Autodesk Inventor part; units mm, degrees
ref_plane "YZ Plane" through (0, 0, 0) normal (1, 0, 0) x (0, 1, 0)
ref_plane "XZ Plane" through (0, 0, 0) normal (0, 1, 0) x (-1, 0, 0)
ref_plane "XY Plane" through (0, 0, 0) normal (0, 0, 1) x (1, 0, 0)
sketch "Sketch1" plane through (0, 0, 0) normal (0, 0, 1) x (1, 0, 0)
  circle A0 centre (0, 0) radius 1.5
  circle A1 centre (47, 0) radius 1.5
  line L0 (1.5, 0) -> (45.5, 0) construction
  circle A2 centre (0, 10) radius 1.5
  circle A3 centre (47, 10) radius 1.5
  line L1 (1.5, 10) -> (45.5, 10) construction
  line L2 (0, 1.5) -> (0, 8.5) construction
  line L3 (47, 1.5) -> (47, 8.5) construction
  line L4 (-5, 30) -> (52, 30)
  line L5 (52, 30) -> (52, -20)
  line L6 (52, -20) -> (-5, -20)
  line L7 (-5, -20) -> (-5, 30)
  line L8 (2.75, 15.25) -> (44.25, 15.25)
  line L9 (44.25, 15.25) -> (44.25, -5.25)
  line L10 (44.25, -5.25) -> (2.75, -5.25)
  line L11 (2.75, -5.25) -> (2.75, 15.25)
  point P0 (23.5, 15.25)
  point P1 (23.5, 30)
  point P2 (44.25, 5)
  point P3 (52, 5)
  point P4 (2.75, 5)
  point P5 (-5, 5)
  point P6 (0, 5)
  dimension "d0" = 3
  dimension "d1" = 3
  dimension "d2" = 44
  dimension "d3" = 3
  dimension "d4" = 3
  dimension "d6" = 7
  dimension "d7" = 5
  dimension "d8" = 5
  dimension "d11" = 20.5
  dimension "d12" = 41.5
  dimension "d22" = 50
extrude "Extrusion1" add sketch "Sketch1" against normal blind 28
sketch "Sketch2" plane through (0, 0, 0) normal (0, 0, 1) x (1, 0, 0)
  line L0 (-5, 30) -> (52, 30)
  line L1 (-5, 30) -> (-26, 30)
  line L2 (-26, 30) -> (-26, -20)
  line L3 (-26, -20) -> (-5, -20)
  line L4 (-5, -20) -> (-5, 30)
  line L5 (2.75, -5.25) -> (2.75, 15.25)
  point P0 (0, 0)
  dimension "d15" = 28.75
extrude "Extrusion2" add sketch "Sketch2" against normal blind 28
sketch "Sketch3" plane through (0, 0, -28) normal (0, 0, -1) x (-1, 0, 0)
  line L0 (-2.75, 15.25) -> (-2.75, -5.25) construction
  line L1 (-2.75, -5.25) -> (-44.25, -5.25) construction
  line L2 (-44.25, -5.25) -> (-44.25, 15.25) construction
  line L3 (-44.25, 15.25) -> (-2.75, 15.25) construction
  circle A0 centre (-47, 10) radius 1.5 construction
  circle A1 centre (0, 10) radius 1.5 construction
  circle A2 centre (-47, 0) radius 1.5 construction
  circle A3 centre (0, 0) radius 1.5 construction
  line L4 (26, 30) -> (-52, 30)
  line L5 (-52, 30) -> (-52, -20)
  line L6 (-52, -20) -> (26, -20)
  line L7 (26, -20) -> (26, 30)
extrude "Extrusion3" add sketch "Sketch3" along normal blind 2
sketch "Sketch5" plane through (0, 0, -30) normal (0, 0, -1) x (-1, 0, 0)
  line L0 (-1, -10) -> (-25, -10) construction
  line L1 (-25, -10) -> (-25, 20) construction
  line L2 (-25, 20) -> (-1, 20) construction
  line L3 (-1, 20) -> (-1, -10) construction
  circle A0 centre (-1, -10) radius 1.5
  circle A1 centre (-25, -10) radius 1.5
  circle A2 centre (-25, 20) radius 1.5
  circle A3 centre (-1, 20) radius 1.5
  line L4 (-52, -20) -> (26, -20)
  line L5 (26, -20) -> (26, 30)
  point P0 (0, 0)
  point P1 (-13, -10)
  point P2 (-1, 5)
  point P3 (26, 5)
  point P4 (-13, -20)
  dimension "d23" = 24
  dimension "d24" = 30
  dimension "d25" = 3
  dimension "d26" = 3
  dimension "d27" = 3
  dimension "d28" = 3
extrude "Extrusion4" cut sketch "Sketch5" against normal blind 20
sketch "Sketch6" plane through (0, 0, 0) normal (0, 0, 1) x (1, 0, 0)
  line L0 (2.75, -5.25) -> (2.75, 15.25)
  line L1 (2.75, 15.25) -> (44.25, 15.25)
  line L2 (44.25, 15.25) -> (44.25, -5.25)
  line L3 (44.25, -5.25) -> (2.75, -5.25)
  circle A0 centre (47, 10) radius 1.5
  circle A1 centre (0, 10) radius 1.5
  circle A2 centre (47, 0) radius 1.5
  circle A3 centre (0, 0) radius 1.5
  line L4 (-26, 30) -> (52, 30)
  line L5 (-26, 30) -> (-26, -20)
  line L6 (52, -20) -> (-26, -20)
  line L7 (52, 30) -> (52, -20)
  line L8 (52, 30) -> (52, -20)
  line L9 (52, 17.25) -> (-5, 17.25)
  line L10 (-5, 17.25) -> (-5, -7.25)
  line L11 (-5, -7.25) -> (52, -7.25)
  line L12 (52, -7.25) -> (52, 17.25)
  point P0 (44.25, 5)
  point P1 (52, 5)
  dimension "d35" = 7.75
  dimension "d36" = 2
extrude "Extrusion5" add sketch "Sketch6" along normal blind 12 contours L4 L7 L9 L10 L11 L6 L5
sketch "Sketch7" plane through (-26, -20, -30) normal (-1, 0, 0) x (0, 0, 1)
  line L0 (42, 0) -> (42, 12.75)
  line L1 (0, 0) -> (0, 50)
  arc A0 (42, 0) -> (0, 0) centre (21, -198.8944) ccw
  line L2 (42, 50) -> (0, 50)
  line L3 (42, 37.25) -> (42, 50)
  arc A1 (0, 50) -> (42, 50) centre (21, 248.8944) ccw
  line L4 (0, 0) -> (42, 0)
  point P0 (30, 20)
  dimension "d39" = 200
  dimension "d40" = 200
extrude "Extrusion6" cut sketch "Sketch7" against normal through all
sketch "Sketch8" plane through (0, 0, 12) normal (0, 0, 1) x (1, 0, 0)
  line L0 (-26, 30) -> (52, 30)
  line L1 (52, -20) -> (-26, -20)
  arc A0 (52, 30) -> (52, -20) centre (250.4313, 5) ccw
  arc A1 (-26, -20) -> (-26, 30) centre (-224.4313, 5) ccw
  line L2 (52, -20) -> (52, 30)
  line L3 (-26, 30) -> (-26, -20)
  line L4 (-26, 28.8944) -> (52, 28.8944)
  point P0 (0, 0)
  dimension "d43" = 200
  dimension "d44" = 200
extrude "Extrusion7" cut sketch "Sketch8" against normal through all contours A1 L4 L3 | L2 L4 A0 | A1 L3 L4 | L4 L2 A0
fillet "Fillet3" radius 10 4 edges at (-25.8638, -18.8944, -9) (-25.8638, 28.8944, -9) (51.8638, -18.8944, -9) (51.8638, 28.8944, -9)
sketch "Sketch9" plane through (2.75, -5.25, 0) normal (1, 0, 0) x (0, 0, -1)
  line L0 (0, 0) -> (0, 20.5) construction
  line L1 (0, 0) -> (28, 0) construction
  line L2 (28, 20.5) -> (28, 0) construction
  line L3 (0, 20.5) -> (28, 20.5) construction
  line L4 (28, 15.25) -> (23, 15.25)
  line L5 (23, 15.25) -> (23, 5.25)
  line L6 (23, 5.25) -> (28, 5.25)
  line L7 (28, 5.25) -> (28, 15.25)
  point P0 (0, 5.25)
  point P1 (28, 10.25)
  dimension "d48" = 5
  dimension "d49" = 10
extrude "Extrusion8" cut sketch "Sketch9" against normal through all
sketch "Sketch10" plane through (0, 0, 0) normal (0, 0, 1) x (1, 0, 0)
  line L0 (2.75, 0) -> (2.75, 10)
  line L1 (2.75, -5.25) -> (2.75, 15.25)
  line L2 (2.75, 8) -> (-2.25, 8)
  line L3 (-2.25, 8) -> (-2.25, 2)
  line L4 (-2.25, 2) -> (2.75, 2)
  line L5 (2.75, 2) -> (2.75, 8)
  point P0 (0, 0)
  point P1 (2.75, 5)
  dimension "d52" = 5
  dimension "d53" = 6
extrude "Extrusion9" cut sketch "Sketch10" against normal blind 28
properties part number "AA048" material "ABS Plastic"
Part model, mm, in its own coordinate system. A direction names the side the tool comes from. Coordinates: 2 decimals unless noted, no trailing zeros. Write each loop counter-clockwise with the first axis right and the second up, starting at its lowest first coordinate (ties: lowest second). Pieces come first, ordered by that corner, then holes.
Item 1: Slice it at C-C (z = -14.5). Count the separate pieces of the cut face and the enclosed holes in it, and give its area (3 significant figures).
Item 2: Slice it at B-B (x = 32). Write the cut outline in (y, z).
Item 3: Pin check, flat tips, straight feed: pin 1 (2 mm diameter, centred on y = 10.5, z = -14.5, fed in from +X); pin 2 (3.5 mm diameter, centred on x = 47.5, y = 10.5, fed in from +Z); pin 3 (9.5 mm diameter, centred on y = 5, z = 4.5, fed in from +X). Stop position of each tip, or through.
Item 4: Mould opens along Y. For faces 1 (the face through (0, 8, -11)), 2 (the face through (14, 5, -30)) say: released by +Y, released by -Y, zero draft, split by the parting line, or undercut.
Item 5: Probe line 1 (X direction, y = 5.5, z = -11.5); line 2 (Y direction, x = 1, z = -24); line 3 (X direction, y = 2.5, z = -18). List the from-to ranges inside material, lowest first.
Item 6: Slice it at A-A (y = 6.5). Write the cut outline in (x, z), and give its area (3 significant figures).
Item 7: Which spindle directions (+Z, -Z, +X, -X, +Y, -Y) get a long thin tool onto all of the face, cutting with end or side? Do faces 3 (the face through (-13, 0, -25)), 4 (the face through (23, -6, 0)), 5 (the face through (4, -11, 12)), 6 (the face through (23, 15.25, -14)), 7 (the face through (1.195, 21.487, -20.14)). Say none if no direction does.
Results found:
1. separate pieces: 1
1. enclosed holes: 9
1. area: 2,590 mm2
2. outline: (-20, -30) - (30, -30) arc R200 cw to (30, 12) - (17.25, 12) - (17.25, 0) - (15.25, 0) - (15.25, -28) - (-5.25, -28) - (-5.25, 0) - (-7.25, 0) - (-7.25, 12) - (-20, 12) arc R200 cw to start
3. pin 1: stops at x = 50.54
3. pin 2: stops at z = 0
3. pin 3: stops at x = 50.44
4. face 1: undercut
4. face 2: zero draft
5. line 1: x = -24.43 to -2.25, 44.25 to 50.43
5. line 2: y = -19.46 to -11.5, -8.5 to -1.12, 11.12 to 18.5, 21.5 to 29.46
5. line 3: x = -24.45 to -2.25, 44.25 to 50.45
6. outline: (-24.44, -30) - (50.44, -30) - (50.44, 0) - (44.25, 0) - (44.25, -28) - (-24.44, -28) - close; (-24.44, -23) - (-2.25, -23) - (-2.25, 0) - (-5, 0) - (-5, 12) - (-24.44, 12) - close
6. area: 1,070 mm2
7. face 3: -X
7. face 4: +Z, +X
7. face 5: +Z, +X, -X, +Y, -Y
7. face 6: +Z
7. face 7: -Z
